```python
from build123d import *

# Parameters (mm, degrees)
F2_R     = 18.6597493024
F3_DEPTH = 163
F4_T     = -2.5


# Not quite as in the source:
# - a fillet or chamfer that OpenCascade refuses, or shapes differently, is made with other operations: its cross-section is extruded or revolved along the edge and cut away or added


with BuildPart() as f1:
    # F0 (on Top) → F1 (revolve)
    with BuildSketch(Plane.XY):
        with BuildLine():
            Line((-80, 0), (80, 0))
            ThreePointArc((80, 0), (0, 80), (-80, 0))
        make_face()
    revolve(axis=Axis((0, 0, 0), (-1, 0, 0)))

    # F2 (on Front) → F3 (join)
    with BuildSketch(Plane.XZ):
        Circle(F2_R)
    extrude(amount=F3_DEPTH)

    # F4
    f4_openings = [f1.faces().sort_by_distance(p)[0] for p in [
        (0, -163, 0),
    ]]
    offset(amount=F4_T, openings=f4_openings, kind=Kind.INTERSECTION)

    # F5: chamfer of 15 on 3 edges, made by hand

    # F5_s1 → F5_t2 (revolve)
    with BuildSketch(Plane.XY):
        with BuildLine():
            Line((28.3450520489, -74.8101465352), (18.6597493072, -88.8370490105))
            Line((18.6597493072, -88.8370490105), (18.6597493024, -77.7934043218))
            ThreePointArc((18.6597493024, -77.7934043218), (23.7757008768, -76.3853130389), (28.3450520489, -74.8101465352))
        make_face()
    revolve(axis=Axis((2.4e-09, -77.7934043218, -1e-10), (0, -1, 0)))

    # F5_s3 → F5_t4 (revolve, cut)
    with BuildSketch(Plane.XY):
        Polygon((18.6597493024, -148), (3.6597493024, -163), (18.6597493024, -163), align=None)
    revolve(axis=Axis((0, -163, 0), (0, -1, 0)), mode=Mode.SUBTRACT)


solid = f1.part
```
Build history of the part. All positions in model axes, mm. Give positions to 0.01 mm unless a question says otherwise; leave off trailing zeros. Loops run counter-clockwise (first coordinate to the right, second up) from the corner with the lowest first, then second, coordinate; pieces in that order, holes last.
Item 1: Slice it at D-D, the plane z = 58.5. List the corners of the cut face in (x, y).
Answers follow:
outline: circle Ø109.14 at (0, 0); hole circle Ø101.67 at (0, 0)
Item 2: Drill centre lines: line 1 (Z direction, x = 0, y = -115); line 2 (Y direction, x = -50, z = -41). Where is each one in solid material? Low to high.
Answers follow:
line 1: z = -18.66 to -16.16, 16.16 to 18.66
line 2: y = -47.11 to -42.72, 42.72 to 47.11
Item 3: Flat gauge pins, fed straight in: pin 1 (5 mm diameter, centred on x = 21.5, y = -13, fed in from -Z); pin 2 (6 mm diameter, centred on x = 13, y = -50, fed in from +Z); pin 3 (4 mm diameter, centred on x = 60.5, z = -43, fed in from -Y). Where does each tip first touch, or does it go through?
Answers follow:
pin 1: stops at z = -76.73
pin 2: stops at z = 63.5
pin 3: stops at y = -34.4
Item 4: Slice it at B-B, the plane z = 0. List the corners of the cut face in (x, y).
Answers follow:
outline: (-28.35, -74.81) - (-18.66, -88.84) - (-18.66, -148) - (-16.16, -150.5) - (-16.16, -75.8) arc R77.5 cw (long way) to (16.16, -75.8) - (16.16, -150.5) - (18.66, -148) - (18.66, -88.84) - (28.35, -74.81) arc R80 ccw (long way) to start
Item 5: Slice it at A-A, the plane x = 0. List the corners of the cut face in (y, z).
Answers follow:
outline: (-150.5, -16.16) - (-148, -18.66) - (-88.84, -18.66) - (-74.81, -28.35) arc R80 ccw (long way) to (-74.81, 28.35) - (-88.84, 18.66) - (-148, 18.66) - (-150.5, 16.16) - (-75.8, 16.16) arc R77.5 cw (long way) to (-75.8, -16.16) - close
Item 6: Slice it at C-C, the plane y = -94.5. List the corners of the cut face in (x, z), and give its area (3 significant figures).
Answers follow:
outline: circle Ø37.32 at (0, 0); hole circle Ø32.32 at (0, 0)
area: 273 mm2
Item 7: Pull direction Z, two halves, no side cores. Call faces 1 (the face through (17.237, -118.004, -7.147)), 2 (the face through (15.4, -112.6, 4.9)): released by +Z, released by -Z, zero draft, split by the parting line, or undercut.
Answers follow:
face 1: split by the parting line
face 2: undercut
